Geometry: see drawing. Coordinates: mm, zero at the bounding-box minimum. Give positions to 0.01 mm unless a question says otherwise; leave off trailing zeros. Loops run counter-clockwise (first coordinate to the right, second up) from the corner with the lowest first, then second, coordinate; pieces in that order, holes last. Notation, with made-up numbers: M 13.25,43.25 L 45.25,43.25 A25 ccw 45.25,78.25 Z; hole C 23.25,-13 d5. An arc over 180 degrees is marked long. Put each result on its own line as item: value.
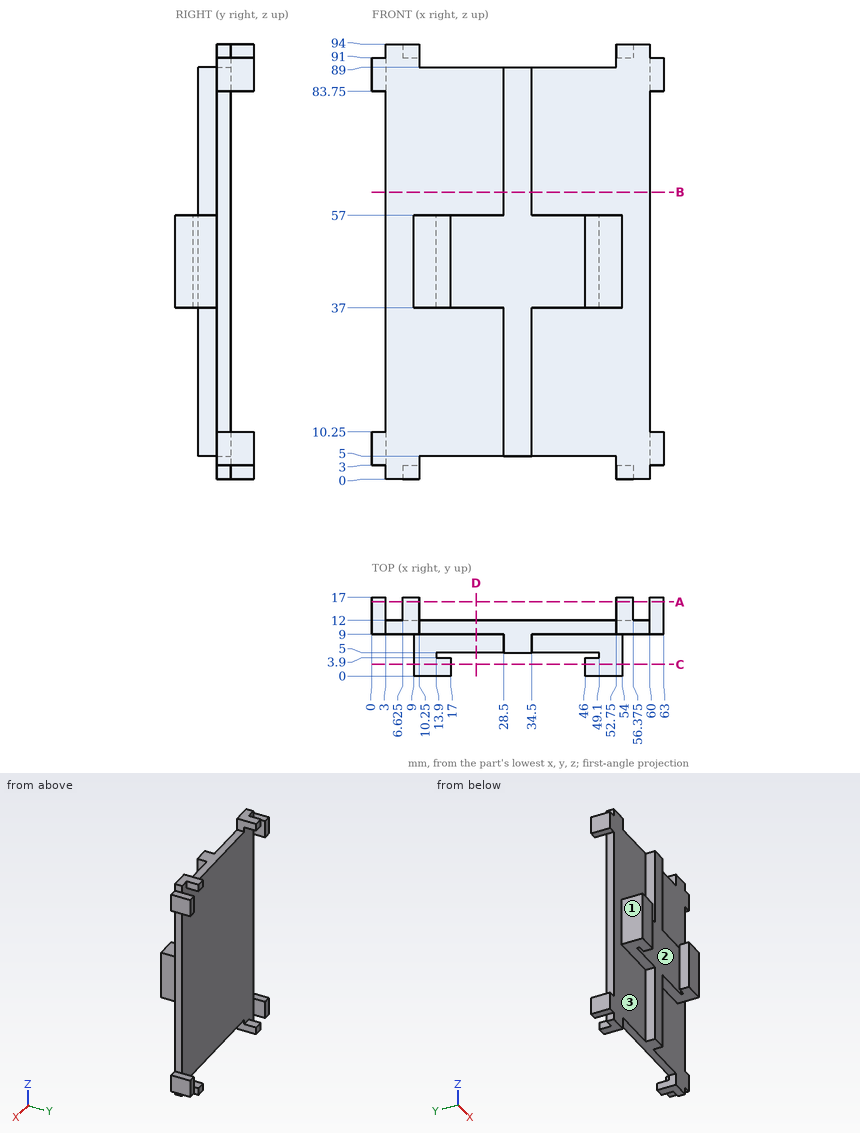
Item 1: Section B-B on z = 62. Output: boundary loops of the cut face in (x, y), then the cut area to 3 significant figures.
Output values:
outline: M 3,9 L 28.5,9 L 28.5,5 L 34.5,5 L 34.5,9 L 60,9 L 60,12 L 3,12 Z
area: 195 mm²
Item 2: Section A-A on y = 16. Count the separate pieces of the cut face and the enclosed holes in it, then the cut area to 4 significant figures.
Output values:
separate pieces: 8
enclosed holes: 0
area: 130.5 mm²
Item 3: Section D-D on x = 22.5. Output: boundary loops of the cut face in (y, z), then the cut area to 3 significant figures.
Output values:
outline: M 5,37 L 9,37 L 9,5 L 12,5 L 12,89 L 9,89 L 9,57 L 5,57 Z
area: 332 mm²
Item 4: Pin query (flat end, axial travel): pin 1 Ø2 at (x, z) = (28.5, 63) entering from -Y; pin 2 Ø0.9 at (x, z) = (15, 45) entering from +Y; pin 3 Ø2.5 at (y, z) = (15, 1.5) entering from -X (3 decimals); pin 4 Ø5 at (y, z) = (15, 31) entering from -X. Return the tip coordinate at first contact, or that it passes through.
Output values:
pin 1: y = 5
pin 2: y = 12
pin 3: x = 6.625
pin 4: through
Item 5: Line query: probe 1 along Y at (x, z) = (18.5, 40); probe 2 along Y at (x, z) = (47.5, 17); probe 3 along X at (y, z) = (16.5, 10). Output: solid intervals per line, ascending. Write a range as [from, to].
Output values:
probe 1: [5, 12]
probe 2: [9, 12]
probe 3: [0, 3], [60, 63]
Item 6: Mould query, pull axis X, two halves, no side actions, for the marked faces 1, 2 and 3. Classes: pulls with the +X half, pulls with the -X half, needs draft (parallel to the pull), parting line crosses it, or undercut.
Output values:
face 1: pulls with the -X half
face 2: undercut
face 3: needs draft
Item 7: Section C-C on y = 2.5. Output: boundary loops of the cut face in (x, z), then the cut area to 3 significant figures.
Output values:
outline: M 9,37 L 17,37 L 17,57 L 9,57 Z; M 46,37 L 54,37 L 54,57 L 46,57 Z
area: 320 mm²
